```python
from build123d import *

# Parameters (mm, degrees)
SKETCH2_R           = 6
BOSS_EXTRUDE1_DEPTH = 5
SKETCH3_R           = 10
BOSS_EXTRUDE2_DEPTH = 5
FILLET1_R           = 12


with BuildPart() as part:
    # Sketch2 → Boss-Extrude1 (new, symmetric)
    with BuildSketch(Plane(origin=(0, 0, 0), x_dir=(1, 0, 0), z_dir=(0, 1, 0))):
        with BuildLine():
            Line((68, -25), (68, 25))
            ThreePointArc((68, 25), (56.032896381, 41.958896227), (36.043982083, 36.367918187))
            ThreePointArc((36.043982083, 36.367918187), (19.637945422, 23.224109156), (-0.720723799, 17.985565246))
            ThreePointArc((-0.720723799, 17.985565246), (-17.99639095, -0.360434168), (0, -18))
            ThreePointArc((0, -18), (19.901005, -22.697990001), (35.6, -35.8))
            ThreePointArc((35.6, -35.8), (55.692099788, -42.076299365), (68, -25))
        make_face()
        with Locations(Location((0, 0, 0), (0, 0, 270))):
            Circle(SKETCH2_R, mode=Mode.SUBTRACT)
        with Locations(Location((50, -25, 0), (0, 0, 270))):
            Circle(SKETCH2_R, mode=Mode.SUBTRACT)
        with Locations(Location((50, 25, 0), (0, 0, 270))):
            Circle(SKETCH2_R, mode=Mode.SUBTRACT)
    extrude(amount=BOSS_EXTRUDE1_DEPTH, both=True)

    # Sketch3 → Boss-Extrude2 (add, symmetric)
    with BuildSketch(Plane.XY):
        with BuildLine():
            Line((12, 5), (122, 5))
            ThreePointArc((122, 5), (142.688818499, -24.481496449), (107.928788897, -33.911564626))
            ThreePointArc((107.928788897, -33.911564626), (70.487228363, -12.449894892), (27.978725812, -5))
            Line((27.978725812, -5), (12, -5))
            Line((12, -5), (12, 5))
        make_face()
        with Locations((122, -17)):
            Circle(SKETCH3_R, mode=Mode.SUBTRACT)
    extrude(amount=BOSS_EXTRUDE2_DEPTH, both=True)

    # Fillet1
    fillet1_edges = [part.edges().sort_by_distance(p)[0] for p in [
        (68, 0, 5),
        (68, 0, -5),
    ]]
    fillet(fillet1_edges, radius=FILLET1_R)


solid = part.part
```
CAD build for the part. Positions are in the model's coordinates, mm. A direction names the side the tool comes from. Round coordinates to 2 decimals unless told otherwise and drop trailing zeros. Write each loop counter-clockwise with the first axis right and the second up, starting at its lowest first coordinate (ties: lowest second). Pieces come first, ordered by that corner, then holes.
Item 1: Band-saw the part on D-D on y = -3. Write the cut outline in (x, z), then the cut area to 3 significant figures.
Filled in:
outline: (-0.72, -17.99) arc R50 cw to (36.04, -36.37) arc R18 ccw to (68, -25) - (68, -17) arc R12 cw to (80, -5) - (138.97, -5) - (138.97, 5) - (80, 5) arc R12 cw to (68, 17) - (68, 25) arc R18 ccw to (35.6, 35.8) arc R44.5 cw to (0, 18) arc R18 ccw to start; hole circle Ø12 at (0, 0); hole circle Ø12 at (50, -25); hole circle Ø12 at (50, 25)
area: 5,210 mm2
Item 2: Band-saw the part on B-B on x = 50. Write the cut outline in (y, z).
Filled in:
outline: (-6.96, -5) - (-5, -5) - (-5, -19) - (5, -19) - (5, 19) - (-5, 19) - (-5, 5) - (-6.96, 5) - close; (-5, -43) - (5, -43) - (5, -31) - (-5, -31) - close; (-5, 31) - (5, 31) - (5, 43) - (-5, 43) - close
Item 3: Mould opens along Z. For faces 4 (the cylindrical face through (114.63, -10.24, -0.07)), 5 (the cylindrical face through (71.42, 0.07, -8.61)), 6 (the cylindrical face through (50, 0, 19)) say: released by +Z, released by -Z, zero draft, split by the parting line, or undercut.
Filled in:
face 4: zero draft
face 5: released by -Z
face 6: undercut
Item 4: Band-saw the part on C-C on z = 22. Write the cut outline in (x, y), then the cut area to 3 significant figures.
Filled in:
outline: (18.44, -5) - (44.8, -5) - (44.8, 5) - (18.44, 5) - close; (55.2, -5) - (68, -5) - (68, 5) - (55.2, 5) - close
area: 392 mm2
Item 5: Band-saw the part on A-A on y = -17. Write the cut outline in (x, z), then the cut area to 3 significant figures.
Filled in:
outline: (81.42, -5) - (112, -5) - (112, 5) - (81.42, 5) - close; (132, -5) - (144, -5) - (144, 5) - (132, 5) - close
area: 426 mm2
Item 6: Drill centre lines: L1, parallel to Y at x = 53.5, z = -20; L2, parallel to Y at x = 137, z = 1.5. Where is each one in solid material? Low to high.
Filled in:
L1: y = -5 to 5
L2: y = -33.09 to -0.91
Item 7: Drop flat-ended pins along their axis: pin 1 Ø3 at (x, z) = (25.5, 16) entering from -Y; pin 2 Ø22 at (x, y) = (88.5, -20) entering from -Z; pin 3 Ø11 at (x, z) = (50, 25) entering from -Y; pin 4 Ø6.5 at (y, z) = (1, -20.5) entering from +X. Give the stop position or say it passes through.
Filled in:
pin 1: stops at y = -5
pin 2: stops at z = -5
pin 3: passes through
pin 4: stops at x = 68
Item 8: Tool access for faces 1 (the cylindrical face through (19.64, 0.07, 22.57)), 2 (the flat face through (68, 0, 21)), 3 (the flat face through (68, 0, -21)): list every direction of +Z, -Z, +X, -X, +Y, -Y with a clear straight run to the whole face (end or side of a thin tool).
Filled in:
face 1: +Z, -X, +Y, -Y
face 2: +Z, +X, +Y, -Y
face 3: -Z, +X, +Y, -Y
